Source: CAD feature listing. Evaluate the final solid. Frame: model axes, mm. A direction names the side the tool comes from. Round coordinates to 2 decimals unless told otherwise and drop trailing zeros. Order: outer loops, then holes, each group sorted by start corner. A loop starts at its lowest first (then second) coordinate and runs counter-clockwise, first axis right, second up. Notation, with made-up numbers: (64.5, 10.25) -> (120.5, 10.25) arc R27 cw to (120.5, 44.25) -> close; hole circle Ø10 at (-27.5, -23). An arc over 180 degrees is marked (long way). Use a Markdown table: item, result. Add a question column.
```python
from build123d import *

# Parameters (mm, degrees)
SKETCH3_R               = 8
BOSS_EXTRUDE1_DEPTH     = 46.103684211
CUT_EXTRUDE1_DEPTH      = 13.730251515
CUT_EXTRUDE1_DEPTH_BACK = 13.730251515
BOSS_EXTRUDE2_DEPTH     = 1.2
CUT_EXTRUDE2_DEPTH      = 1.6
SKETCH8_R               = 1.4
SKETCH8_R_2             = 1.6
CUT_EXTRUDE3_DEPTH      = 2.64160469
CUT_EXTRUDE3_DEPTH_BACK = 50.446677335
CUT_EXTRUDE4_DEPTH      = 50.446677335


with BuildPart() as part:
    # Sketch3 → Boss-Extrude1 (new body)
    with BuildSketch(Plane(origin=(-20.344467381, 196.178792599, 0), x_dir=(-0.994665758, -0.103150523, 0), z_dir=(0.103150523, -0.994665758, 0))):
        with Locations((-10.431405186, 0)):
            Circle(SKETCH3_R)
    extrude(amount=BOSS_EXTRUDE1_DEPTH)

    # Sketch4 → Cut-Extrude1 (cut, two sides)
    with BuildSketch(Plane(origin=(10.375761543, 1.076004901, 0), x_dir=(0.103150523, -0.994665758, 0), z_dir=(-0.994665758, -0.103150523, 0))) as cut_extrude1_sk:
        Polygon((-197.230869842, 0), (-189.230869842, 8), (-197.230869842, 8), align=None)
        Polygon((-159.127185631, 8), (-151.127185631, 8), (-151.127185631, 0), align=None)
    extrude(amount=CUT_EXTRUDE1_DEPTH, mode=Mode.SUBTRACT)
    extrude(cut_extrude1_sk.sketch, amount=-CUT_EXTRUDE1_DEPTH_BACK, mode=Mode.SUBTRACT)

    # Sketch5 → Boss-Extrude2 (add, symmetric)
    with BuildSketch(Plane(origin=(10.375761543, 1.076004901, 0), x_dir=(0.103150523, -0.994665758, 0), z_dir=(-0.994665758, -0.103150523, 0))):
        with BuildLine():
            Line((-151.127185631, -2.8), (-148.702314501, 1.4))
            ThreePointArc((-148.702314501, 1.4), (-150.761712293, 2.776045612), (-153.107084619, 1.979898987))
            Line((-153.107084619, 1.979898987), (-151.127185631, 0))
            Line((-151.127185631, 0), (-151.127185631, -2.8))
        make_face()
    extrude(amount=BOSS_EXTRUDE2_DEPTH, both=True)

    # Sketch7 → Cut-Extrude2 (cut, symmetric)
    with BuildSketch(Plane(origin=(10.375761543, 1.076004901, 0), x_dir=(0.103150523, -0.994665758, 0), z_dir=(-0.994665758, -0.103150523, 0))):
        with BuildLine():
            Line((-194.968128142, 2.2627417), (-197.230869842, 0))
            Line((-197.230869842, 0), (-197.230869842, -3.2))
            ThreePointArc((-197.230869842, -3.2), (-194.274455338, -1.224586984), (-194.968128142, 2.2627417))
        make_face()
    extrude(amount=CUT_EXTRUDE2_DEPTH, both=True, mode=Mode.SUBTRACT)

    # Sketch8 → Cut-Extrude3 (cut, two sides)
    with BuildSketch(Plane(origin=(-20.344467381, 196.178792599, 0), x_dir=(0.994665758, 0.103150523, 0), z_dir=(-0.103150523, 0.994665758, 0))) as cut_extrude3_sk:
        with Locations((10.431405186, -5.5)):
            Circle(SKETCH8_R)
        with Locations((6.831405186, 3)):
            Circle(SKETCH8_R_2)
        with Locations((14.031405186, 3)):
            Circle(SKETCH8_R_2)
    extrude(amount=CUT_EXTRUDE3_DEPTH, mode=Mode.SUBTRACT)
    extrude(cut_extrude3_sk.sketch, amount=-CUT_EXTRUDE3_DEPTH_BACK, mode=Mode.SUBTRACT)

    # Sketch9 → Cut-Extrude4 (cut, through all)
    with BuildSketch(Plane(origin=(-20.344467381, 196.178792599, 0), x_dir=(0.994665758, 0.103150523, 0), z_dir=(-0.103150523, 0.994665758, 0))):
        with BuildLine():
            Line((7.933405986, 7.6), (12.929404385, 7.6))
            ThreePointArc((12.929404385, 7.6), (10.431405186, 8), (7.933405986, 7.6))
        make_face()
        with BuildLine():
            Line((7.933405986, -7.6), (12.929404385, -7.6))
            ThreePointArc((12.929404385, -7.6), (10.431405186, -8), (7.933405986, -7.6))
        make_face()
    extrude(amount=-CUT_EXTRUDE4_DEPTH, mode=Mode.SUBTRACT)


solid = part.part
```
1) Section C-C on z = -5.5. Output: boundary loops of the cut face in (x, y).
2) Line query: probe 1 along X at (y, z) = (162, -3); probe 2 along Z at (x, y) = (-8.5, 183.5); probe 3 along Z at (x, y) = (-4.5, 152). Output: solid intervals per line, ascending. Write a range as from..to.
3) First-contact query: pin 1 Ø1 at (x, y) = (-12, 155.5) entering from +Z; pin 2 Ø8 at (y, z) = (184.5, -5) entering from -X; pin 3 Ø8 at (x, y) = (-0.5, 179.5) entering from -Z. Flat tips, straight axial feed; report the tip coordinate or a pass-through.
4) Section B-B on y = 187.5. Count the separate pieces of the cut face and the enclosed holes in it, then the cut area to 3 significant figures.
5) Reachability of faces 4 (the flat face through (-11.397, 195.521, -0.43)), 5 (the flat face through (-6.387, 151.083, 0.661)), 6 (the flat face through (-9.78, 194.36, 2.9)), 7 (the flat face through (-4, 151.33, 0.66)), 8 (the flat face through (-8.215, 195.851, -0.43)) from +Z, -Z, +X, -X, +Y, -Y: full face, straight path, thin tool, end or side. Return the list, or none.
6) Draft query along Z for faces 1 (the cylindrical face through (-7.8, 174.59, 4.11)), 2 (the flat face through (-8, 175, -7.6)), 3 (the cylindrical face through (0.332, 175.472, -0.14)). Return one class per face: pulls with the +Z half, pulls with the -Z half, needs draft (parallel to the pull), parting line crosses it, or undercut.
7) Section A-A on z = 5. Output: boundary loops of the cut face in (x, y), then the cut area to 3 significant figures.
Conclusion:
| question | item | result |
|---|---|---|
| 1 | outline | (-15.75, 196.66) -> (-10.99, 150.8) -> (0.57, 152) -> (-4.19, 197.85) -> close |
| 2 | probe 1 | x = -13.77..-11.54, -8.32..-4.3, -1.08..1.14 |
| 2 | probe 2 | z = -7.6..4.1, 6.9..7.6 |
| 2 | probe 3 | z = -7.6..2.75 |
| 3 | pin 1 | stops at z = 5.21 |
| 3 | pin 2 | stops at x = -16.75 |
| 3 | pin 3 | stops at z = -7.15 |
| 4 | separate pieces | 1 |
| 4 | enclosed holes | 3 |
| 4 | area | 177 mm^2 |
| 5 | face 4 | +Y |
| 5 | face 5 | +Z, -Y |
| 5 | face 6 | +Z, -X, +Y |
| 5 | face 7 | +Z, +X |
| 5 | face 8 | none |
| 6 | face 1 | undercut |
| 6 | face 2 | pulls with the -Z half |
| 6 | face 3 | parting line crosses it |
| 7 | outline | (-15.66, 191.64) -> (-11.94, 155.73) -> (-7.03, 156.24) -> (-10.75, 192.15) -> close; (-8.15, 192.42) -> (-4.43, 156.51) -> (0.48, 157.01) -> (-3.24, 192.93) -> close |
| 7 | area | 357 mm^2 |
